Design review of the part built by this model. Coordinates are the model's own, in mm. A direction names the side the tool comes from. Round coordinates to 2 decimals unless told otherwise and drop trailing zeros. Order: outer loops, then holes, each group sorted by start corner. A loop starts at its lowest first (then second) coordinate and runs counter-clockwise, first axis right, second up. Notation, with made-up numbers: (8.25, -14.5) - (59.25, -14.5) arc R14 ccw to (59.25, -2.5) - close; hole circle Ø5 at (44.5, 88.5). An arc over 180 degrees is marked (long way). Write item = value, one per line.
from build123d import *

# Parameters (mm, degrees)
SKETCH1_W               = 38.1
SKETCH1_H               = 38.1
SKETCH1_W_2             = 31.75
SKETCH1_H_2             = 31.75
BOSS_EXTRUDE1_DEPTH     = 192.0875
FILLET1_R               = 3.81
FILLET2_R               = 0.635
SKETCH2_R               = 2.65
CUT_EXTRUDE1_DEPTH      = 20.05
CUT_EXTRUDE1_DEPTH_BACK = 20.05


with BuildPart() as part:
    # Sketch1 → Boss-Extrude1 (new body, symmetric)
    with BuildSketch(Plane.XY):
        Rectangle(SKETCH1_W, SKETCH1_H)
        Rectangle(SKETCH1_W_2, SKETCH1_H_2, mode=Mode.SUBTRACT)
    extrude(amount=BOSS_EXTRUDE1_DEPTH, both=True)

    # Fillet1
    fillet1_edges = [part.edges().sort_by_distance(p)[0] for p in [
        (19.05, -19.05, 0),
        (-19.05, -19.05, 0),
        (-19.05, 19.05, 0),
        (19.05, 19.05, 0),
    ]]
    fillet(fillet1_edges, radius=FILLET1_R)

    # Fillet2
    fillet2_edges = [part.edges().sort_by_distance(p)[0] for p in [
        (15.875, -15.875, 0),
        (15.875, 15.875, 0),
        (-15.875, 15.875, 0),
        (-15.875, -15.875, 0),
    ]]
    fillet(fillet2_edges, radius=FILLET2_R)

    # Sketch2 → Cut-Extrude1 (cut, two sides)
    with BuildSketch(Plane(origin=(0, 0, 0), x_dir=(0, 0, -1), z_dir=(1, 0, 0))) as cut_extrude1_sk:
        with Locations((-180, 0)):
            Circle(SKETCH2_R)
        with Locations((-120, 0)):
            Circle(SKETCH2_R)
        with Locations((-60, 0)):
            Circle(SKETCH2_R)
        Circle(SKETCH2_R)
        with Locations((60, 0)):
            Circle(SKETCH2_R)
        with Locations((120, 0)):
            Circle(SKETCH2_R)
        with Locations((180, 0)):
            Circle(SKETCH2_R)
    extrude(amount=CUT_EXTRUDE1_DEPTH, mode=Mode.SUBTRACT)
    extrude(cut_extrude1_sk.sketch, amount=-CUT_EXTRUDE1_DEPTH_BACK, mode=Mode.SUBTRACT)


solid = part.part
1) The part is to be moulded in two halves that separate along Y. For faces 1 (the flat face through (0, -15.875, 3)), 2 (the flat face through (19.05, 0, 3)), 3 (the flat face through (0, -19.05, 3)), say which applies: released by +Y, released by -Y, zero draft, split by the parting line, or undercut.
Findings:
face_1 = undercut
face_2 = zero draft
face_3 = released by -Y
2) To check wall thickness, follow L1, parallel to Y at x = -5.5, z = -155.5 (3 decimals); L2, parallel to Y at x = 18, z = -120. State the ranges of each line that lie inside material, in increasing order. Write a range as from..to.
Findings:
L1 = -19.05..-15.875, 15.875..19.05
L2 = -17.87..-2.65, 2.65..17.87
3) For faces 4 (the flat face through (-17, 0, 192.088)), 5 (the flat face through (-15.875, 0, 3)), list the 3-axis set-ups (+Z, -Z, +X, -X, +Y, -Y) from which the entire face can be reached by the end or side of a thin tool; tool diameter is ignored.
Findings:
face_4 = +Z, +X, -X, +Y, -Y
face_5 = +Z, -Z
4) We need section A-A on z = 74.5. Write out the cut boundary in (x, y) (3 decimals).
Findings:
outline = (-19.05, -15.24) arc R3.81 ccw to (-15.24, -19.05) - (15.24, -19.05) arc R3.81 ccw to (19.05, -15.24) - (19.05, 15.24) arc R3.81 ccw to (15.24, 19.05) - (-15.24, 19.05) arc R3.81 ccw to (-19.05, 15.24) - close; hole (-15.875, -15.24) arc R0.635 ccw to (-15.24, -15.875) - (15.24, -15.875) arc R0.635 ccw to (15.875, -15.24) - (15.875, 15.24) arc R0.635 ccw to (15.24, 15.875) - (-15.24, 15.875) arc R0.635 ccw to (-15.875, 15.24) - close
